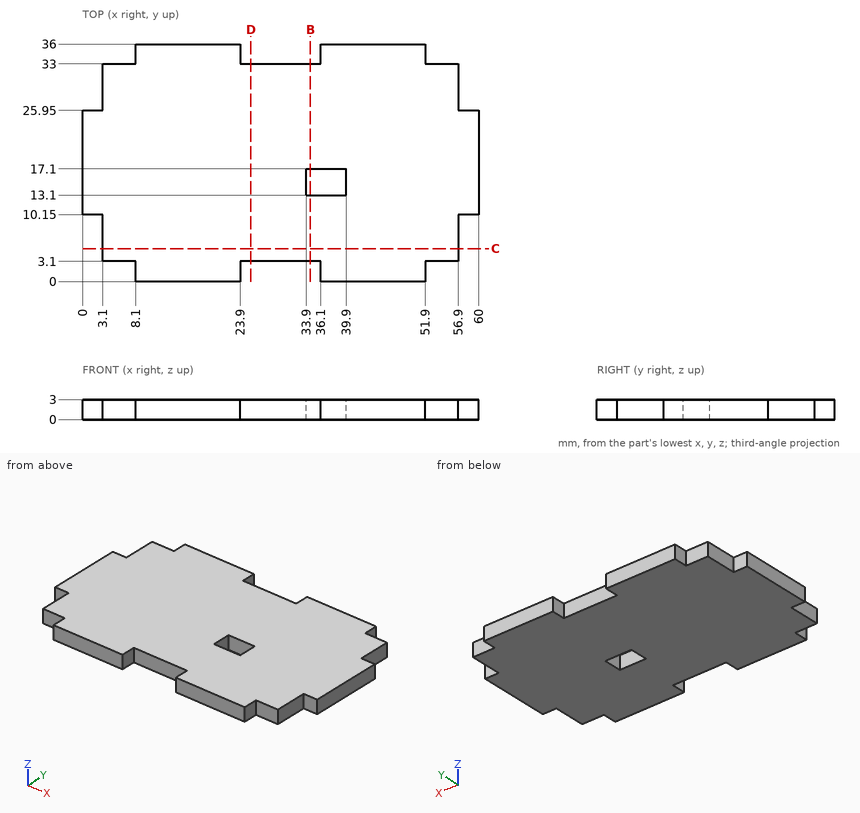
Drawing for the job (mm, zero at the part's lowest x, y, z). Round coordinates to 2 decimals unless told otherwise and drop trailing zeros. Loops run counter-clockwise (first coordinate to the right, second up) from the corner with the lowest first, then second, coordinate; pieces in that order, holes last. Notation, with made-up numbers: (3, 21) - (43, 21) arc R21 ccw to (43, 26) - close; hole circle Ø11 at (-5.5, 61.25). An arc over 180 degrees is marked (long way). Return JSON: item names as keys, results as strings. Group by question number.
Q1. Band-saw the part on D-D on x = 25.5. Give the cut face in (y, z), plus the area to 3 significant figures.
Q2. Band-saw the part on B-B on x = 34.5. Give the cut face in (y, z).
Q3. Drill centre lines: line 1 along Y through (x, z) = (35, 2.45); line 2 along X through (y, z) = (16, 2.45); line 3 along Y through (x, z) = (26, 1.2). Where is each one in solid material? Low to high. Write a range as [from, to].
Q4. Band-saw the part on C-C on y = 5. Give the cut face in (x, z).
Q5. Flat gauge pins, fed straight in: pin 1 Ø0.9 at (y, z) = (1, 2) entering from -X; pin 2 Ø1.5 at (y, z) = (9, 1.5) entering from +X; pin 3 Ø0.9 at (x, z) = (1, 1.5) entering from +Y. Where does each tip first touch, or does it go through?
Solutions:
{
 "1": {"outline": "(3.1, 0) - (33, 0) - (33, 3) - (3.1, 3) - close", "area": "89.7 mm^2"},
 "2": {"outline": "(3.1, 0) - (13.1, 0) - (13.1, 3) - (3.1, 3) - close; (17.1, 0) - (33, 0) - (33, 3) - (17.1, 3) - close"},
 "3": {"line 1": "y = [3.1, 13.1], [17.1, 33]", "line 2": "x = [0, 33.9], [39.9, 60]", "line 3": "y = [3.1, 33]"},
 "4": {"outline": "(3.1, 0) - (56.9, 0) - (56.9, 3) - (3.1, 3) - close"},
 "5": {"pin 1": "stops at x = 8.1", "pin 2": "stops at x = 56.9", "pin 3": "stops at y = 25.95"}
}
